For this review, take the finished solid that the model builds, in its own axes (mm). Face numbers are marked on the shaded views. A direction names the side the tool comes from. Round coordinates to 2 decimals unless told otherwise and drop trailing zeros. Write each loop counter-clockwise with the first axis right and the second up, starting at its lowest first coordinate (ties: lowest second). Pieces come first, ordered by that corner, then holes. Notation, with made-up numbers: M 30.5,-33.5 L 69.5,-33.5 A34 ccw 69.5,4.5 Z; hole C 13.25,-23.75 d3. An arc over 180 degrees is marked long. Answer in a Markdown table with one row per item.
```python
from build123d import *

# Parameters (mm, degrees)
F1_DEPTH      = 17.54
F1_DEPTH_BACK = 9.92
F0_W          = 2
F0_H          = 2
F2_DEPTH      = 1
F4_DEPTH      = 10
F6_DEPTH      = 10


with BuildPart() as f1:
    # F0 (on Front) → F1 (new body, two sides)
    with BuildSketch(Plane.XZ) as f1_sk:
        Polygon((7.4, 8.065), (-7.4, 8.065), (-7.4, 6.065), (-7.4, -6.065), (-7.4, -8.065), (7.4, -8.065), (7.4, -6.065), (7.4, 6.065), align=None)
    extrude(amount=F1_DEPTH)
    extrude(f1_sk.sketch, amount=-F1_DEPTH_BACK)

    # F0 (on Front) → F2 (join)
    with BuildSketch(Plane.XZ):
        with Locations((-8.4, 7.065)):
            Rectangle(F0_W, F0_H)
        with Locations((-8.4, -7.065)):
            Rectangle(F0_W, F0_H)
        with Locations((8.4, -7.065)):
            Rectangle(F0_W, F0_H)
        with Locations((8.4, 7.065)):
            Rectangle(F0_W, F0_H)
    extrude(amount=F2_DEPTH)

    # F3 (on face) → F4 (cut)
    with BuildSketch(Plane.XZ.offset(17.54)):
        Polygon((-5.75, -3.950203), (0, -3.950203), (5.75, -3.950203), (5.75, 2.549797), (3, 2.549797), (3, 4.049797), (0, 4.049797), (-3, 4.049797), (-3, 2.549797), (-5.75, 2.549797), align=None)
    extrude(amount=-F4_DEPTH, mode=Mode.SUBTRACT)

    # F5 (on face) → F6 (cut)
    with BuildSketch(Plane(origin=(0, 9.92, 0), x_dir=(-1, 0, 0), z_dir=(0, 1, 0))):
        Polygon((-5.668929, -3.996807), (0.081071, -3.996807), (5.831071, -3.996807), (5.831071, 2.503193), (3.081071, 2.503193), (3.081071, 4.003193), (0.081071, 4.003193), (-2.918929, 4.003193), (-2.918929, 2.503193), (-5.668929, 2.503193), align=None)
    extrude(amount=-F6_DEPTH, mode=Mode.SUBTRACT)


solid = f1.part
```
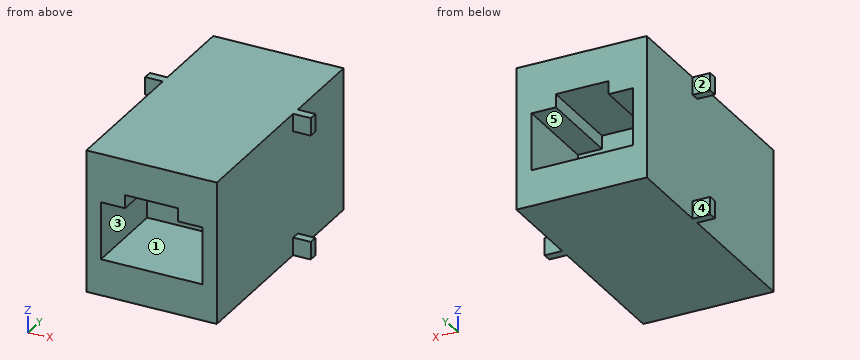
Q1. Take a section at C-C (z = 1). State the section outline as (x, y) points, then the cut area to 3 significant figures.
Found:
| item | result |
|---|---|
| outline | M -7.4,-17.54 L -5.75,-17.54 L -5.75,-7.54 L 5.75,-7.54 L 5.75,-17.54 L 7.4,-17.54 L 7.4,9.92 L 5.67,9.92 L 5.67,-0.08 L -5.83,-0.08 L -5.83,9.92 L -7.4,9.92 Z |
| area | 176 mm² |
Q2. Insertion check: P1, Ø1.6, axis at x = -8.5, z = -7.5, coming from the +Y side; P2, Ø4, axis at y = 5, z = -6, coming from the -X side; P3, Ø0.6, axis at x = 8.5, z = -7, coming from the -Y side; P4, Ø6, axis at x = 1, z = 2, coming from the -Y side. Each pin has a flat end and moves straight along its axis. Give the tip position at first contact, or say it passes through.
Found:
| item | result |
|---|---|
| P1 | y = 0 |
| P2 | x = -7.4 |
| P3 | y = -1 |
| P4 | y = -17.54 |
Q3. Mouldability with a two-part tool opening along X and no side actions: class the marked faces 1 and 2 as +X half, -X half, draft (parallel to the pull), parting line (faces both ways), or undercut.
Found:
| item | result |
|---|---|
| face 1 | undercut |
| face 2 | draft |
Q4. Take a section at A-A (y = 8.25). State the section outline as (x, z) points (3 decimals).
Found:
| item | result |
|---|---|
| outline | M -7.4,-8.065 L 7.4,-8.065 L 7.4,8.065 L -7.4,8.065 Z; hole M -5.831,-3.997 L 5.669,-3.997 L 5.669,2.503 L 2.919,2.503 L 2.919,4.003 L -3.081,4.003 L -3.081,2.503 L -5.831,2.503 Z |
Q5. Take a section at B-B (x = 1.25). State the section outline as (y, z) points (3 decimals), then the cut area to 3 significant figures.
Found:
| item | result |
|---|---|
| outline | M -17.54,-8.065 L 9.92,-8.065 L 9.92,-3.997 L -0.08,-3.997 L -0.08,4.003 L 9.92,4.003 L 9.92,8.065 L -17.54,8.065 L -17.54,4.05 L -7.54,4.05 L -7.54,-3.95 L -17.54,-3.95 Z |
| area | 283 mm² |
Q6. Machinability: for the marked faces 3, 4 and 5, which of the approach directions +Z, -Z, +X, -X, +Y, -Y give a long, thin tool a straight path to every point of the face, cutting with its end or side? Answer none if there is none.
Found:
| item | result |
|---|---|
| face 3 | -Y |
| face 4 | +Z, -Z, -X, +Y |
| face 5 | +Y |
Q7. For probe 1 along X at (y, z) = (6, 1.25); probe 2 along Z at (x, y) = (-1, 6.5) (3 decimals); probe 3 along Z at (x, y) = (3, 6.25) (3 decimals), list the stretches that pass through material, from the lowest coordinate up.
Found:
| item | result |
|---|---|
| probe 1 | -7.4 to -5.83, 5.67 to 7.4 |
| probe 2 | -8.065 to -3.997, 4.003 to 8.065 |
| probe 3 | -8.065 to -3.997, 2.503 to 8.065 |
Q8. Take a section at D-D (y = -5). State the section outline as (x, z) points (3 decimals), then the cut area to 3 significant figures.
Found:
| item | result |
|---|---|
| outline | M -7.4,-8.065 L 7.4,-8.065 L 7.4,8.065 L -7.4,8.065 Z |
| area | 239 mm² |
